Could you check a few things on this model? Use its own coordinates, in mm. Round coordinates to 2 decimals unless told otherwise and drop trailing zeros. Loops run counter-clockwise (first coordinate to the right, second up) from the corner with the lowest first, then second, coordinate; pieces in that order, holes last. Notation, with made-up numbers: (66, 86.25) -> (106, 86.25) arc R7 ccw to (106, 97.25) -> close; hole circle Ø7 at (8.25, -38.75). An arc over 180 degrees is marked (long way). Write each question's results on one line, items separated by ' | '. Start each with the question number.
1) For P1, Ø0.8, axis at x = -2.54, y = 0, coming from the -Z side, with a flat end and sliding along its axis, tell me the tip position at first contact or that it passes through.
2) Imagine slicing it at A-A, the plane y = 0. List the corners of the cut face in (x, z) for me (3 decimals), plus the area to 3 significant figures.
3) Imagine slicing it at C-C, the plane x = -4.75. List the corners of the cut face in (y, z) for me (3 decimals), plus the area to 3 significant figures.
4) Imagine slicing it at B-B, the plane x = 0. List the corners of the cut face in (y, z) for me (3 decimals), plus the area to 3 significant figures.
from build123d import *

# Parameters (mm, degrees)
SKETCH002_W            = 15.24
SKETCH002_H            = 2
PAD001_DEPTH           = 0.035
SKETCH003_R            = 0.51
POCKET001_DEPTH        = 0.036
LINEARPATTERN004_COUNT = 7
LINEARPATTERN004_PITCH = 2.54


with BuildPart() as part:
    # Sketch002 → Pad001 (new body)
    with BuildSketch(Plane.XY):
        Rectangle(SKETCH002_W, SKETCH002_H)
    extrude(amount=-PAD001_DEPTH)

    # Sketch003 → Pocket001 (cut, through all)
    with BuildSketch(Plane.XY):
        with Locations((-7.62, 0)):
            Circle(SKETCH003_R)
    pocket001 = extrude(amount=-POCKET001_DEPTH, mode=Mode.SUBTRACT)

    # LinearPattern004: Pocket001 ×7
    with Locations(*[(i * LINEARPATTERN004_PITCH, 0, 0) for i in range(1, LINEARPATTERN004_COUNT)]):
        add(pocket001, mode=Mode.SUBTRACT)


solid = part.part
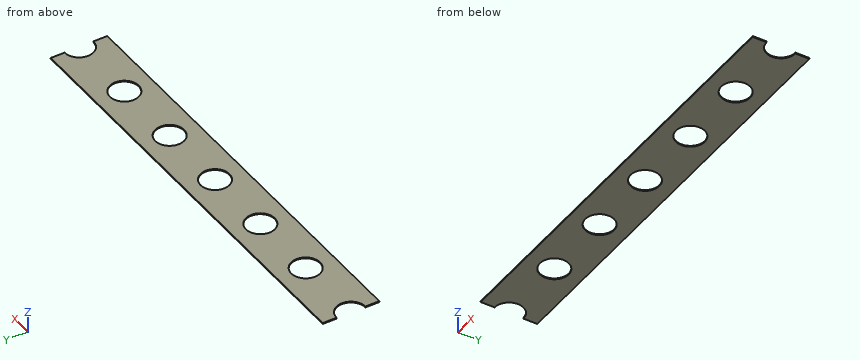
Checked values:
1) P1: through
2) outline: (-7.11, -0.035) -> (-5.59, -0.035) -> (-5.59, 0) -> (-7.11, 0) -> close; (-4.57, -0.035) -> (-3.05, -0.035) -> (-3.05, 0) -> (-4.57, 0) -> close; (-2.03, -0.035) -> (-0.51, -0.035) -> (-0.51, 0) -> (-2.03, 0) -> close; (0.51, -0.035) -> (2.03, -0.035) -> (2.03, 0) -> (0.51, 0) -> close; (3.05, -0.035) -> (4.57, -0.035) -> (4.57, 0) -> (3.05, 0) -> close; (5.59, -0.035) -> (7.11, -0.035) -> (7.11, 0) -> (5.59, 0) -> close | area: 0.319 mm^2
3) outline: (-1, -0.035) -> (-0.389, -0.035) -> (-0.389, 0) -> (-1, 0) -> close; (0.389, -0.035) -> (1, -0.035) -> (1, 0) -> (0.389, 0) -> close | area: 0.0428 mm^2
4) outline: (-1, -0.035) -> (-0.51, -0.035) -> (-0.51, 0) -> (-1, 0) -> close; (0.51, -0.035) -> (1, -0.035) -> (1, 0) -> (0.51, 0) -> close | area: 0.0343 mm^2
